Part model, mm, in its own coordinate system. Face numbers are marked on the shaded views. A direction names the side the tool comes from. Coordinates: 2 decimals unless noted, no trailing zeros. Write each loop counter-clockwise with the first axis right and the second up, starting at its lowest first coordinate (ties: lowest second). Pieces come first, ordered by that corner, then holes. Notation, with made-up numbers: (63, 81.5) -> (107, 81.5) arc R29 cw to (107, 115.5) -> close; hole circle Ø11 at (52.5, -24). An arc over 180 degrees is marked (long way). One line per question, with ' | ' between items. Start each with the question number.
Item 1: Saw through at D-D (z = 9.5). List the corners of the cut face in (x, y).
Item 2: 3-axis set-ups, long thin cutter, end or side, ignore diameter. For the marked faces 1 and 2: which of +Z, -Z, +X, -X, +Y, -Y reach the whole face in a straight line?
Item 3: Saw through at A-A (z = 0). List the corners of the cut face in (x, y), and give its area (3 significant figures).
Item 4: Pin check, flat tips, straight feed: pin 1 (4 mm diameter, centred on x = 1, z = 1, fed in from +Y); pin 2 (4 mm diameter, centred on x = 1, z = -5.5, fed in from -Y); pin 3 (4 mm diameter, centred on x = 0, y = 4, fed in from +Z); pin 4 (1.5 mm diameter, centred on x = -2.5, y = 2, fed in from -Z). Stop position of each tip, or through.
Item 5: Saw through at C-C (x = 1). List the corners of the cut face in (y, z), and give its area (3 significant figures).
Item 6: Two-plate mould, pull along Y, no slides. Class the marked faces 3 and 4: pulls with the +Y half, pulls with the -Y half, needs draft (parallel to the pull), parting line crosses it, or undercut.
Item 7: Probe probe 1 along Y at (x, z) = (3.75, 0); probe 2 along Y at (x, z) = (-2.95, 0); probe 3 along Z at (x, y) = (3.75, -3.5). List the from-to ranges inside material, lowest first. Write a range as [from, to].
from build123d import *


with BuildPart() as part:
    # Sketch1 → Revolve1 (revolve)
    with BuildSketch(Plane.XY, mode=Mode.PRIVATE) as revolve1_sk:
        Polygon((0, 5), (4.5, 5), (4.5, 7.5), (3.5, 7.5), (3.5, 12.5), (4.5, 12.5), (4.5, 15), (0, 15), align=None)
    revolve1 = revolve(revolve1_sk.sketch.rotate(Axis((-243.027564124, 0, 0), (1, 0, 0)), 90), axis=Axis((-243.027564124, 0, 0), (1, 0, 0)))

    # Mirror1: Revolve1 across Right Plane
    add(revolve1.mirror(Plane(origin=(0, 0, 0), x_dir=(0, 0, -1), z_dir=(1, 0, 0))))


solid = part.part
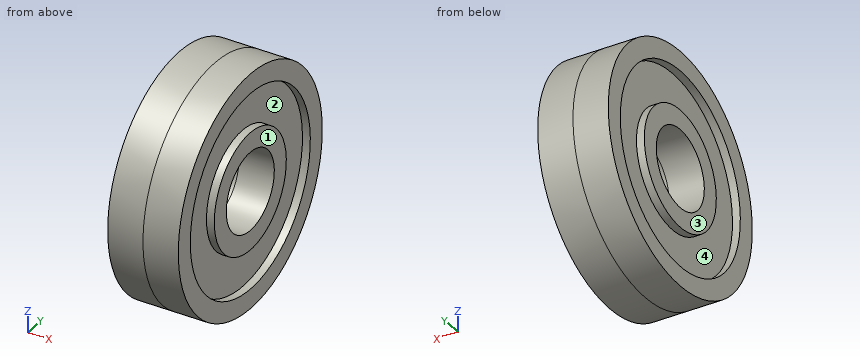
From the geometry:
1) outline: (-4.5, -11.61) -> (4.5, -11.61) -> (4.5, -8.12) -> (3.5, -8.12) -> (3.5, 8.12) -> (4.5, 8.12) -> (4.5, 11.61) -> (-4.5, 11.61) -> (-4.5, 8.12) -> (-3.5, 8.12) -> (-3.5, -8.12) -> (-4.5, -8.12) -> close
2) face 1: +Z, -Z, +X, +Y, -Y | face 2: +X
3) outline: (-4.5, -15) -> (4.5, -15) -> (4.5, -12.5) -> (3.5, -12.5) -> (3.5, -7.5) -> (4.5, -7.5) -> (4.5, -5) -> (-4.5, -5) -> (-4.5, -7.5) -> (-3.5, -7.5) -> (-3.5, -12.5) -> (-4.5, -12.5) -> close; (-4.5, 5) -> (4.5, 5) -> (4.5, 7.5) -> (3.5, 7.5) -> (3.5, 12.5) -> (4.5, 12.5) -> (4.5, 15) -> (-4.5, 15) -> (-4.5, 12.5) -> (-3.5, 12.5) -> (-3.5, 7.5) -> (-4.5, 7.5) -> close | area: 160 mm2
4) pin 1: y = 15 | pin 2: y = -14.59 | pin 3: z = 14.87 | pin 4: z = -14.95
5) outline: circle Ø30 at (0, 0); hole circle Ø10 at (0, 0) | area: 628 mm2
6) face 3: needs draft | face 4: undercut
7) probe 1: [-15, -12.5], [-7.5, -5], [5, 7.5], [12.5, 15] | probe 2: [-15, -5], [5, 15] | probe 3: [-14.59, -12], [-6.63, -3.57], [3.57, 6.63], [12, 14.59]
